The drawing under review shows one solid part. Ordinate dimensions are in mm from its lowest x, y, z. A direction names the side the tool comes from. Coordinates: 2 decimals unless noted, no trailing zeros. Write each loop counter-clockwise with the first axis right and the second up, starting at its lowest first coordinate (ties: lowest second). Pieces come first, ordered by that corner, then holes.
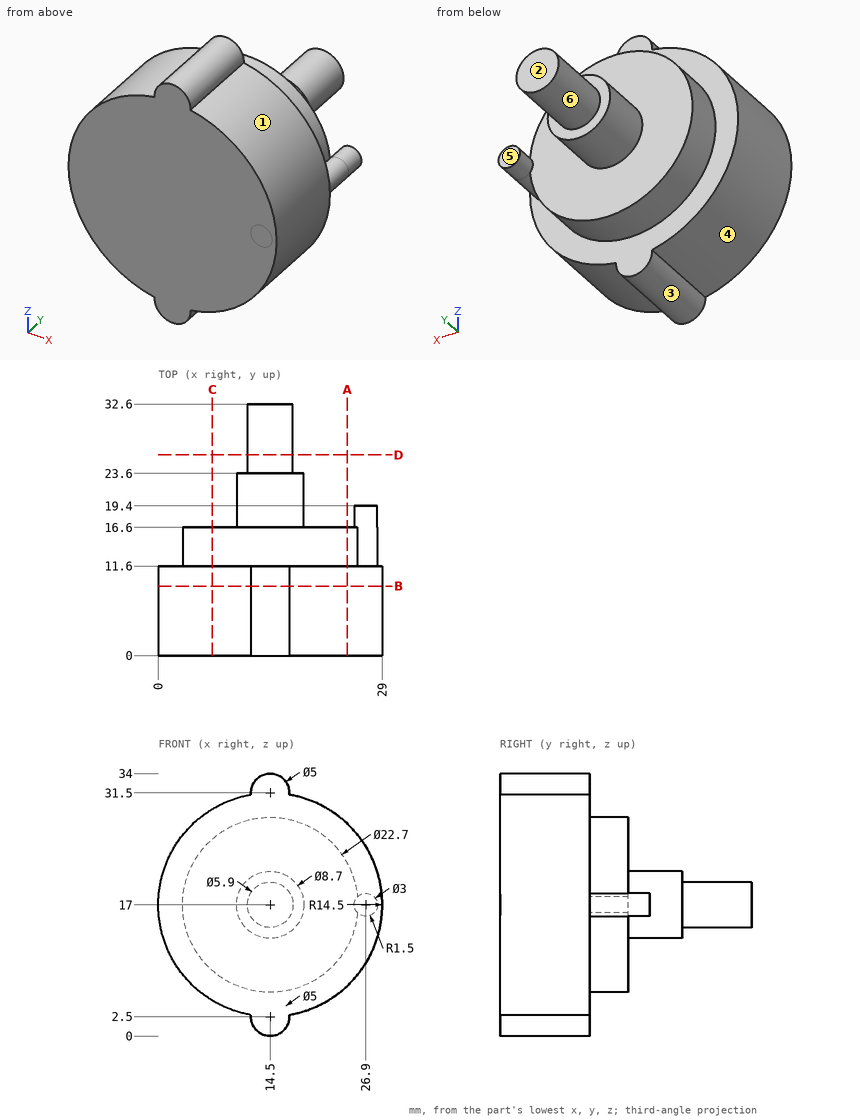
1) For L1, parallel to Y at x = 10, z = 19.5; L2, parallel to Y at x = 24.5, z = 11.5; L3, parallel to X at y = 10.5, z = 28.5, list the stretches that pass through material, from the lowest coordinate up.
2) Consider section B-B (y = 9). Give the boundary of the cut face in (x, z), then the cut area to 3 significant figures.
3) Tool access review of the marked faces 4, 5 and 6: name each direction out of +Z, -Z, +X, -X, +Y, -Y from which nothing blocks a thin tool from reaching the whole face with its end or side.
4) Consider section A-A (x = 24.5). Give the boundary of the cut face in (y, z).
5) Consider section D-D (y = 26). Give the boundary of the cut face in (x, z).
6) The part is to be moulded in two halves that separate along X. For the marked faces 1, 2 and 3, say which applies: pulls with the +X half, pulls with the -X half, needs draft (parallel to the pull), parting line crosses it, or undercut.
7) Consider section C-C (x = 7). Give the boundary of the cut face in (y, z).
8) Clearance check with flat-ended pins moving along their axes: P1, Ø6, axis at x = 22, y = 4, coming from the +Z side; P2, Ø10, axis at x = 9, z = 24, coming from the +Y side; P3, Ø10, axis at x = 14, y = 25.5, coming from the -Z side. State where each tip first meets the part, or that it passes through.
Results:
1. L1: y = 0 to 16.6
1. L2: y = 0 to 11.6
1. L3: x = 5.67 to 23.33
2. outline: (12.01, 2.72) arc R2.5 ccw (long way) to (16.99, 2.72) arc R14.5 ccw to (16.99, 31.28) arc R2.5 ccw (long way) to (12.01, 31.28) arc R14.5 ccw to start
2. area: 681 mm2
3. face 4: -X, +Y, -Y
3. face 5: +Z, -Z, +X, +Y
3. face 6: +Y
4. outline: (0, 6.5) - (11.6, 6.5) - (11.6, 11.63) - (16.6, 11.63) - (16.6, 22.37) - (11.6, 22.37) - (11.6, 27.5) - (0, 27.5) - close
5. outline: circle Ø5.9 at (14.5, 17)
6. face 1: pulls with the +X half
6. face 2: needs draft
6. face 3: parting line crosses it
7. outline: (0, 4.59) - (11.6, 4.59) - (11.6, 8.48) - (16.6, 8.48) - (16.6, 25.52) - (11.6, 25.52) - (11.6, 29.41) - (0, 29.41) - close
8. P1: stops at z = 30.78
8. P2: stops at y = 23.6
8. P3: stops at z = 12.65
